Verification items for this drawing (mm, ordinates from the low corner). Round coordinates to 2 decimals unless told otherwise and drop trailing zeros. Order: outer loops, then holes, each group sorted by start corner. A loop starts at its lowest first (then second) coordinate and runs counter-clockwise, first axis right, second up. Notation, with made-up numbers: (61.5, 18.25) -> (91.5, 18.25) arc R19 cw to (91.5, 42.25) -> close; hole circle Ø4 at (-29.75, 81.5). An arc over 180 degrees is marked (long way). Answer in a Markdown table with one row per item.
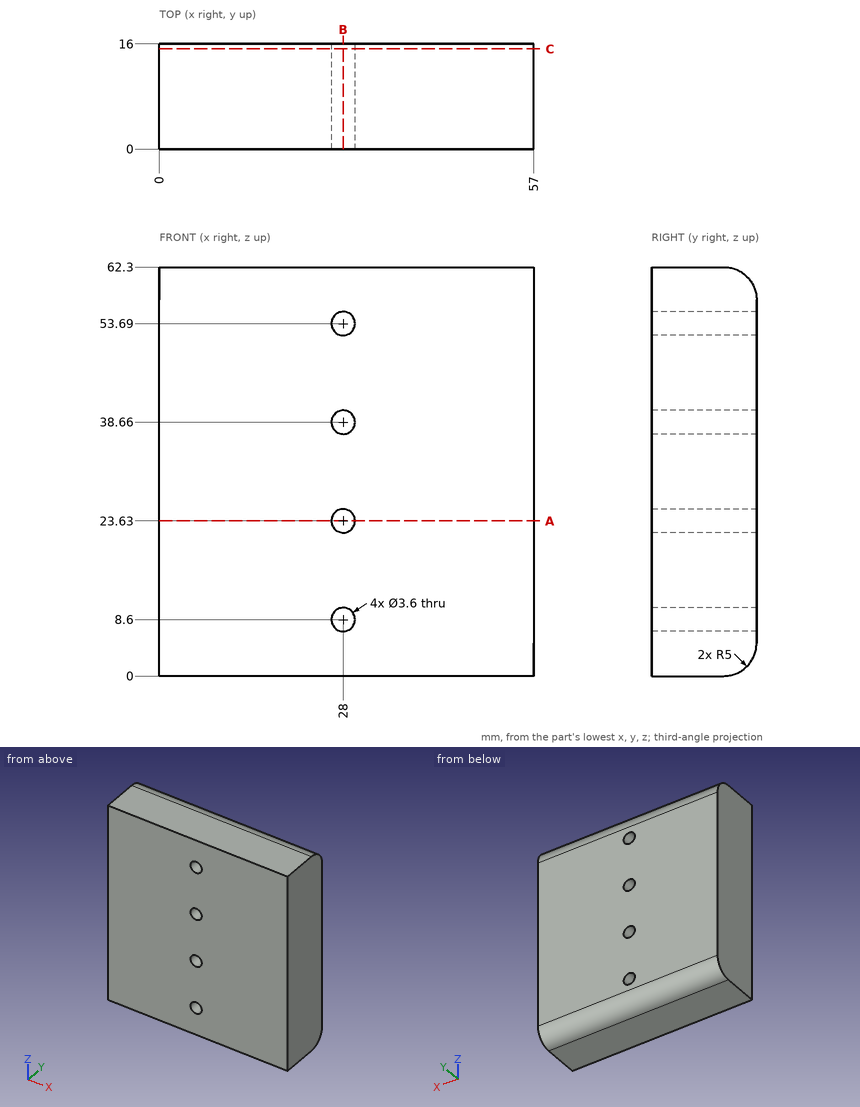
Item 1: Depth check by flat-ended pin: P1, Ø3, axis at x = 28, z = 53.69, coming from the -Y side. Enter the tip coordinate at first touch or a pass-through.
Result sheet:
| item | result |
|---|---|
| P1 | passes through |
Item 2: Cross-section at B-B (x = 28). Record the boundary of the cut face in (y, z).
Result sheet:
| item | result |
|---|---|
| outline | (0, 0) -> (11, 0) arc R5 ccw to (16, 5) -> (16, 6.8) -> (0, 6.8) -> close; (0, 10.4) -> (16, 10.4) -> (16, 21.83) -> (0, 21.83) -> close; (0, 25.43) -> (16, 25.43) -> (16, 36.86) -> (0, 36.86) -> close; (0, 40.46) -> (16, 40.46) -> (16, 51.89) -> (0, 51.89) -> close; (0, 55.49) -> (16, 55.49) -> (16, 57.3) arc R5 ccw to (11, 62.3) -> (0, 62.3) -> close |
Item 3: Cross-section at C-C (y = 15.25). Record the boundary of the cut face in (x, z), and give its area (3 significant figures).
Result sheet:
| item | result |
|---|---|
| outline | (0, 2.37) -> (57, 2.37) -> (57, 59.93) -> (0, 59.93) -> close; hole circle Ø3.6 at (28, 8.6); hole circle Ø3.6 at (28, 23.63); hole circle Ø3.6 at (28, 38.66); hole circle Ø3.6 at (28, 53.69) |
| area | 3,240 mm^2 |
Item 4: Scan lines: line 1 (Z direction, x = 28, y = 6); line 2 (Z direction, x = 28, y = 12.5); line 3 (X direction, y = 7.75, z = 24.5). Record each from-to range of solid material in increasing order. Write a range as [from, to].
Result sheet:
| item | result |
|---|---|
| line 1 | z = [0, 6.8], [10.4, 21.83], [25.43, 36.86], [40.46, 51.89], [55.49, 62.3] |
| line 2 | z = [0.23, 6.8], [10.4, 21.83], [25.43, 36.86], [40.46, 51.89], [55.49, 62.07] |
| line 3 | x = [0, 26.42], [29.58, 57] |
Item 5: Cross-section at A-A (z = 23.63). Record the boundary of the cut face in (x, y).
Result sheet:
| item | result |
|---|---|
| outline | (0, 0) -> (26.2, 0) -> (26.2, 16) -> (0, 16) -> close; (29.8, 0) -> (57, 0) -> (57, 16) -> (29.8, 16) -> close |
